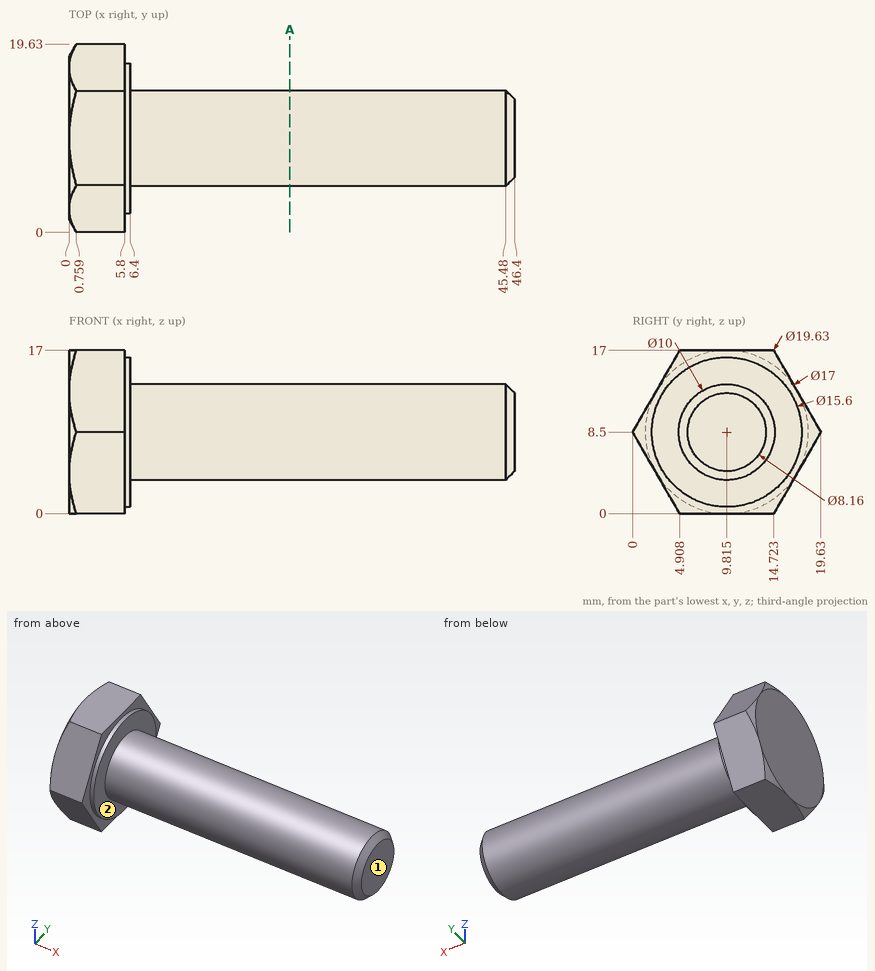
For this review, use the dimensioned drawing (mm, ordinates from the lowest corner) and the shaded views. A direction names the side the tool comes from. Round coordinates to 2 decimals unless told otherwise and drop trailing zeros. Write each loop counter-clockwise with the first axis right and the second up, starting at its lowest first coordinate (ties: lowest second). Pieces come first, ordered by that corner, then holes. Notation, with made-up numbers: (-27.75, -29.75) -> (25.25, -29.75) arc R20 cw to (25.25, -21.75) -> close; hole circle Ø2 at (29, 40.25). An arc over 180 degrees is marked (long way). Answer in a Markdown table with one row per item.
Q1. Clearance check with flat-ended pins moving along their axes: pin 1 Ø1 at (y, z) = (8.5, 14.5) entering from +X; pin 2 Ø2 at (y, z) = (17.5, 15) entering from +X; pin 3 Ø10 at (x, z) = (12, 5) entering from -Y (1 decimal); pin 4 Ø2 at (x, y) = (27.5, 6) entering from +Z. State where each tip first meets the part, or that it passes through.
The answers:
| item | result |
|---|---|
| pin 1 | x = 6.4 |
| pin 2 | through |
| pin 3 | y = 4.8 |
| pin 4 | z = 12.63 |
Q2. Take a section at A-A, the plane x = 23. State the section outline as (y, z) points (1 decimal).
The answers:
| item | result |
|---|---|
| outline | circle Ø10 at (9.8, 8.5) |
Q3. To check wall thickness, follow L1, parallel to X at y = 16.25, z = 5.25; L2, parallel to X at y = 18, z = 10; L3, parallel to Z at x = 30, y = 9.5. State the ranges of each line that lie inside material, in increasing order. Write a range as [from, to].
The answers:
| item | result |
|---|---|
| L1 | [0, 6.4] |
| L2 | [0, 5.8] |
| L3 | [3.51, 13.49] |
Q4. For the marked faces 1 and 2, list the 3-axis set-ups (+Z, -Z, +X, -X, +Y, -Y) from which the entire face can be reached by the end or side of a thin tool; tool diameter is ignored.
The answers:
| item | result |
|---|---|
| face 1 | +Z, -Z, +X, +Y, -Y |
| face 2 | +X |
